Here's how the part is built. I have some questions about the finished solid (model axes, mm). A direction names the side the tool comes from. Round coordinates to 2 decimals unless told otherwise and drop trailing zeros. Write each loop counter-clockwise with the first axis right and the second up, starting at its lowest first coordinate (ties: lowest second). Pieces come first, ordered by that corner, then holes. Notation, with made-up numbers: (81.5, 11.5) - (87.5, 11.5) arc R28 ccw to (87.5, 50.5) - close; hole circle Ø2 at (-36.75, 75.5). An arc over 180 degrees is marked (long way). Use one line per item in the form item = value. Start each with the question number.
1. Will these pins go through, and if not, where does the flat tip stop? pin 1 (1.5 mm diameter, centred on y = 8.5, z = 1, fed in from -X); pin 2 (15 mm diameter, centred on x = 95, z = -2.5, fed in from -Y); pin 3 (16 mm diameter, centred on x = 101, y = 3, fed in from -Z); pin 4 (16 mm diameter, centred on x = 102.5, y = 0, fed in from +Z).
2. Which directions (+Z, -Z, +X, -X, +Y, -Y) give clear straight access to the entire face, cutting with the end or side of a thin tool? Please do faces 1 (the flat face through (100, 0, 27)), 2 (the flat face through (100, 0, -27)), 3 (the flat face through (100.21, -12.214, -22.078)).
3. I want a section at B-B, the plane y = -13.5. List the corners of the cut face in (x, z) for me.
4. I want a section at A-A, the plane x = 73.5. List the corners of the cut face in (y, z) for me, plus the area to 4 significant figures.
5. If I drill on line 1 along Y through (x, z) = (102, 4.5); line 2 along Z through (x, y) = (107, 4.5); line 3 along Y through (x, z) = (21.5, -22.5), over which ranges is the centre line in solid material (lowest first)?
```python
from build123d import *

# Parameters (mm, degrees)
BOSS_EXTRUDE1_DEPTH = 115
CUT_EXTRUDE1_DEPTH  = 30


with BuildPart() as part:
    # Sketch1 → Boss-Extrude1 (new body)
    with BuildSketch(Plane(origin=(0, 0, 0), x_dir=(0, 0, -1), z_dir=(1, 0, 0))):
        Polygon((-17.5, 17.5), (-27.5, 7.5), (-27.5, -7.5), (-17.5, -17.5), (17.5, -17.5), (27.5, -7.5), (27.5, 7.5), (17.5, 17.5), align=None)
    extrude(amount=BOSS_EXTRUDE1_DEPTH)

    # Sketch2 → Cut-Extrude1 (cut)
    with BuildSketch(Plane(origin=(115, 0, 0), x_dir=(0, 0, -1), z_dir=(1, 0, 0))):
        Polygon((27.5, 7.5), (17.5, 17.5), (-17.5, 17.5), (-27.5, 7.5), (-27.5, -7.5), (-17.5, -17.5), (17.5, -17.5), (27.5, -7.5), align=None)
        Polygon((27, 7.292893219), (17.292893219, 17), (-17.292893219, 17), (-27, 7.292893219), (-27, -7.292893219), (-17.292893219, -17), (17.292893219, -17), (27, -7.292893219), align=None, mode=Mode.SUBTRACT)
    extrude(amount=-CUT_EXTRUDE1_DEPTH, mode=Mode.SUBTRACT)


solid = part.part
```
Model answer:
q1.pin_1 = 0
q1.pin_2 = -17
q1.pin_3 = -27
q1.pin_4 = 27
q2.face_1 = +Z, +X, +Y, -Y
q2.face_2 = -Z, +X, +Y, -Y
q2.face_3 = -Z, +X, -Y
q3.outline = (0, -21.5) - (85, -21.5) - (85, -20.79) - (115, -20.79) - (115, 20.79) - (85, 20.79) - (85, 21.5) - (0, 21.5) - close
q4.outline = (-17.5, -17.5) - (-7.5, -27.5) - (7.5, -27.5) - (17.5, -17.5) - (17.5, 17.5) - (7.5, 27.5) - (-7.5, 27.5) - (-17.5, 17.5) - close
q4.area = 1,725 mm2
q5.line_1 = -17 to 17
q5.line_2 = -27 to 27
q5.line_3 = -12.5 to 12.5
